Check sheet for the drawn part. Datum: minimum x, y, z corner. Units: mm. A direction names the side the tool comes from. Round coordinates to 2 decimals unless told otherwise and drop trailing zeros. Order: outer loops, then holes, each group sorted by start corner. A loop starts at its lowest first (then second) coordinate and runs counter-clockwise, first axis right, second up. Notation, with made-up numbers: (79, 18) -> (138, 18) arc R35 cw to (138, 52) -> close; hole circle Ø5 at (-24, 21). An arc over 180 degrees is marked (long way). Use CSV: the item, a comma, the result in double quotes.
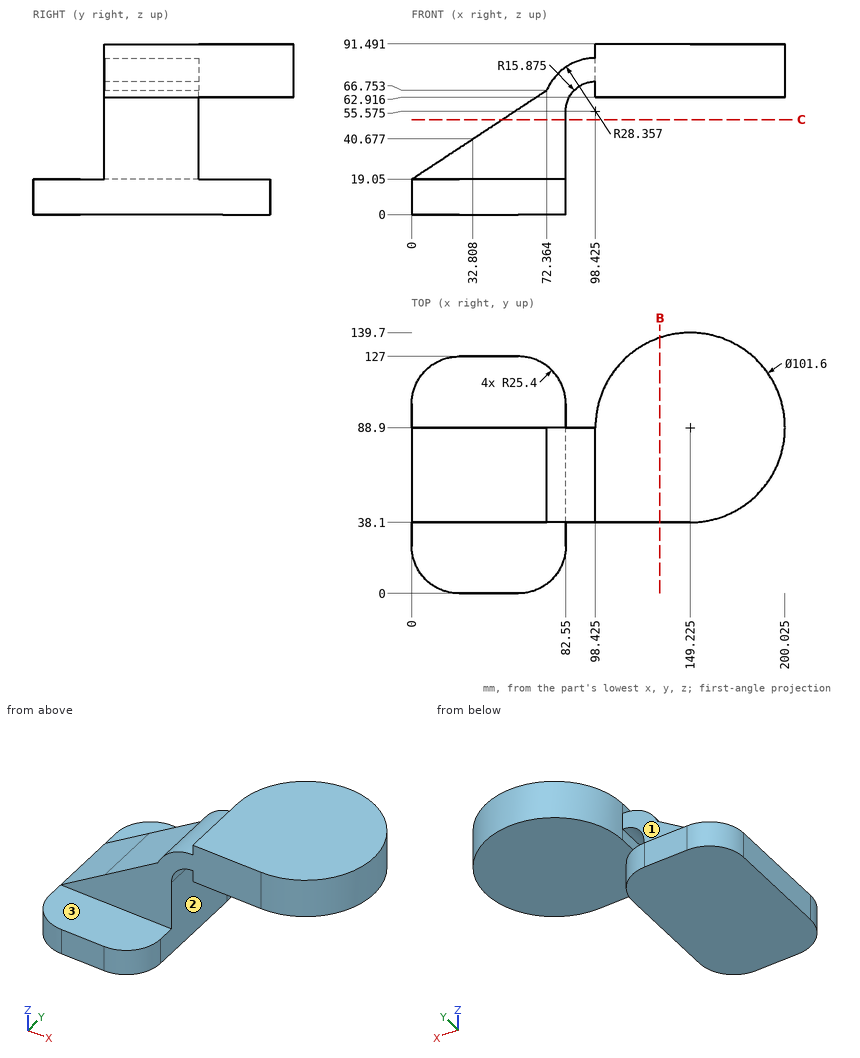
Q1. Access from +Z, -Z, +X, -X, +Y, -Y to the whole of each face (thin tool, end or side, straight path). Record for the marked faces 1, 2 and 3.
Result sheet:
face 1,"+Z, -X, +Y"
face 2,"-Z, +X, +Y, -Y"
face 3,"+Z, +X, -X, -Y"
Q2. Scan lines: L1, parallel to X at y = 71.5, z = 17; L2, parallel to Z at x = 129, y = 54 (1 decimal); L3, parallel to Y at x = 44, z = 34. Record each from-to range of solid material in increasing order.
Result sheet:
L1,"x = 0 to 82.55"
L2,"z = 62.9 to 91.5"
L3,"y = 38.1 to 88.9"
Q3. Sectioned sample at C-C, the plane z = 51. Enter the section's corners in (x, y), then the cut area to 3 significant figures.
Result sheet:
outline,"(48.47, 38.1) -> (82.55, 38.1) -> (82.55, 88.9) -> (48.47, 88.9) -> close"
area,"1,730 mm^2"
Q4. Sectioned sample at B-B, the plane x = 133. Enter the section's corners in (y, z) (1 decimal), then the cut area to 3 significant figures.
Result sheet:
outline,"(38.1, 62.9) -> (137, 62.9) -> (137, 91.5) -> (38.1, 91.5) -> close"
area,"2,830 mm^2"
Q5. Go/stop test with flat-tipped pins: pin 1 (5.5 mm diameter, centred on x = 37, z = 9.5, fed in from +Y); pin 2 (4 mm diameter, centred on y = 72.5, z = 37, fed in from -X) (1 decimal); pin 3 (12 mm diameter, centred on y = 107, z = 65, fed in from -X). Record where each tip stops, or that it passes through.
Result sheet:
pin 1,"stops at y = 127"
pin 2,"stops at x = 24.2"
pin 3,"stops at x = 99.89"
